Check sheet for the modelled part. Datum: model origin and axes. Units: mm. Give positions to 0.01 mm unless a question says otherwise; leave off trailing zeros. Loops run counter-clockwise (first coordinate to the right, second up) from the corner with the lowest first, then second, coordinate; pieces in that order, holes last. Notation, with made-up numbers: (-25, -17) - (11, -17) arc R25 cw to (11, -4) - close; hole circle Ø9 at (56, 59.5). An arc over 180 degrees is marked (long way). Use one line per item in the form item = value.
from build123d import *

# Parameters (mm, degrees)
F0_W     = 115
F0_H     = 65
F1_DEPTH = 3
F2_R     = 2.1
F3_DEPTH = 25
F4_R     = 4
F5_SIZE2 = 0.2886751346
F5_SIZE  = 0.5


with BuildPart() as f1:
    # F0 (on Top) → F1 (new body)
    with BuildSketch(Plane.XY):
        Rectangle(F0_W, F0_H)
        with BuildLine():
            Line((44, -10.5), (-44, -10.5))
            ThreePointArc((-44, -10.5), (-51, -3.5), (-44, 3.5))
            Line((-44, 3.5), (44, 3.5))
            ThreePointArc((44, 3.5), (51, -3.5), (44, -10.5))
        make_face(mode=Mode.SUBTRACT)
    extrude(amount=F1_DEPTH)

    # F2 (on face) → F3 (cut)
    with BuildSketch(Plane.XY.offset(3)):
        with Locations((-36, -21.5)):
            Circle(F2_R)
        with Locations((36, -21.5)):
            Circle(F2_R)
        with Locations((36, 12.5)):
            Circle(F2_R)
        with Locations((-36, 12.5)):
            Circle(F2_R)
    extrude(amount=-F3_DEPTH, mode=Mode.SUBTRACT)

    # F4
    f4_edges = [f1.edges().sort_by_distance(p)[0] for p in [
        (57.5, 32.5, 1.5),
        (-57.5, 32.5, 1.5),
    ]]
    fillet(f4_edges, radius=F4_R)

    # F5
    f5_edges = [f1.edges().sort_by_distance(p)[0] for p in [
        (0, 3.5, 3),
        (0, 3.5, 0),
    ]]
    f5_side = f1.faces().sort_by_distance((0, 3.5, 1.5))[0]
    chamfer(f5_edges, length=F5_SIZE, length2=F5_SIZE2, reference=f5_side)


solid = f1.part
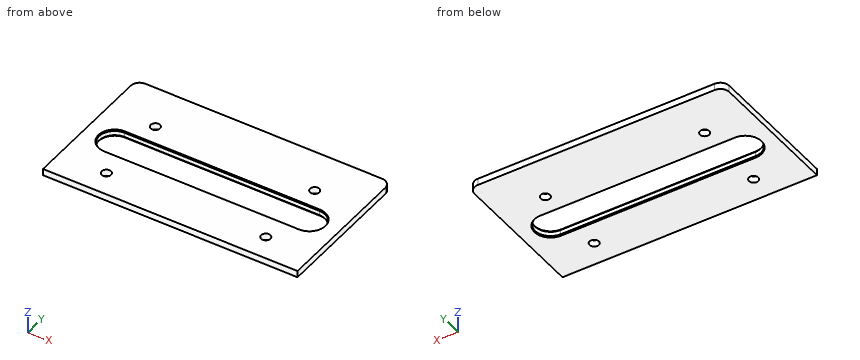
Item 1: Thickness scan on L1, parallel to Y at x = -36, z = 1.15; L2, parallel to X at y = 12, z = 1.4; L3, parallel to Y at x = 36.5, z = 1.05. Record the ranges inside material, lowest first.
Answer block:
L1 = -32.5 to -23.6, -19.4 to -10.5, 3.5 to 10.4, 14.6 to 32.5
L2 = -57.5 to -38.04, -33.96 to 33.96, 38.04 to 57.5
L3 = -32.5 to -23.54, -19.46 to -10.5, 3.5 to 10.46, 14.54 to 32.5
Item 2: Section check D-D on z = 1.1. Record the boundary of the cut face in (x, y), then the cut area to 3 significant figures.
Answer block:
outline = (-57.5, -32.5) - (57.5, -32.5) - (57.5, 28.5) arc R4 ccw to (53.5, 32.5) - (-53.5, 32.5) arc R4 ccw to (-57.5, 28.5) - close; hole (-44, -10.5) - (44, -10.5) arc R7 ccw to (44, 3.5) - (-44, 3.5) arc R7 ccw to start; hole circle Ø4.2 at (-36, -21.5); hole circle Ø4.2 at (-36, 12.5); hole circle Ø4.2 at (36, -21.5); hole circle Ø4.2 at (36, 12.5)
area = 6,030 mm2
Item 3: Section check C-C on y = -21.5. Record the boundary of the cut face in (x, z), then the cut area to 3 significant figures.
Answer block:
outline = (-57.5, 0) - (-38.1, 0) - (-38.1, 3) - (-57.5, 3) - close; (-33.9, 0) - (33.9, 0) - (33.9, 3) - (-33.9, 3) - close; (38.1, 0) - (57.5, 0) - (57.5, 3) - (38.1, 3) - close
area = 320 mm2
Item 4: Section check B-B on x = -36. Record the boundary of the cut face in (y, z).
Answer block:
outline = (-32.5, 0) - (-23.6, 0) - (-23.6, 3) - (-32.5, 3) - close; (-19.4, 0) - (-10.79, 0) - (-10.5, 0.5) - (-10.5, 2.5) - (-10.79, 3) - (-19.4, 3) - close; (3.5, 0.5) - (3.79, 0) - (10.4, 0) - (10.4, 3) - (3.79, 3) - (3.5, 2.5) - close; (14.6, 0) - (32.5, 0) - (32.5, 3) - (14.6, 3) - close
Item 5: Section check A-A on y = -3.5. Record the boundary of the cut face in (x, z).
Answer block:
outline = (-57.5, 0) - (-51.29, 0) - (-51, 0.5) - (-51, 2.5) - (-51.29, 3) - (-57.5, 3) - close; (51, 0.5) - (51.29, 0) - (57.5, 0) - (57.5, 3) - (51.29, 3) - (51, 2.5) - close
